For this review, use the dimensioned drawing (mm, ordinates from the lowest corner) and the shaded views. A direction names the side the tool comes from. Coordinates: 2 decimals unless noted, no trailing zeros. Loops run counter-clockwise (first coordinate to the right, second up) from the corner with the lowest first, then second, coordinate; pieces in that order, holes last. Notation, with made-up numbers: (30, 15.5) - (40, 15.5) arc R28 cw to (40, 44.5) - close; hole circle Ø11 at (-24, 68). An arc over 180 degrees is marked (long way). Use a Markdown table: item, result. Add a question column.
1) Add section A-A, the plane z = 11.5. Give the boundary of the cut face in (x, y), and give its area (3 significant figures).
2) Add section D-D, the plane z = 29. Give the boundary of the cut face in (x, y) (3 decimals).
3) The part is to be moulded in two halves that separate along Y. For the marked faces 1, 2, 3 and 4, say which applies: pulls with the +Y half, pulls with the -Y half, needs draft (parallel to the pull), parting line crosses it, or undercut.
4) Clearance check with a flat-ended pin moving along its axis: pin 1 (1.6 mm diameter, centred on x = 25.5, y = 119.5, fed in from +Z). State where the tip first meets the part, or that it passes through.
5) Add section B-B, the plane y = 100.4. Give the boundary of the cut face in (x, z).
6) To check wall thickness, follow L1, parallel to Y at x = 60.5, z = 12; L2, parallel to Z at x = 185, y = 113. State the ranges of each line that lie inside material, in increasing order. Write a range as [from, to].
7) Add section C-C, the plane x = 112.7. Give the boundary of the cut face in (y, z) (3 decimals).
8) For the marked faces 5 and 6, list the 3-axis set-ups (+Z, -Z, +X, -X, +Y, -Y) from which the entire face can be reached by the end or side of a thin tool; tool diameter is ignored.
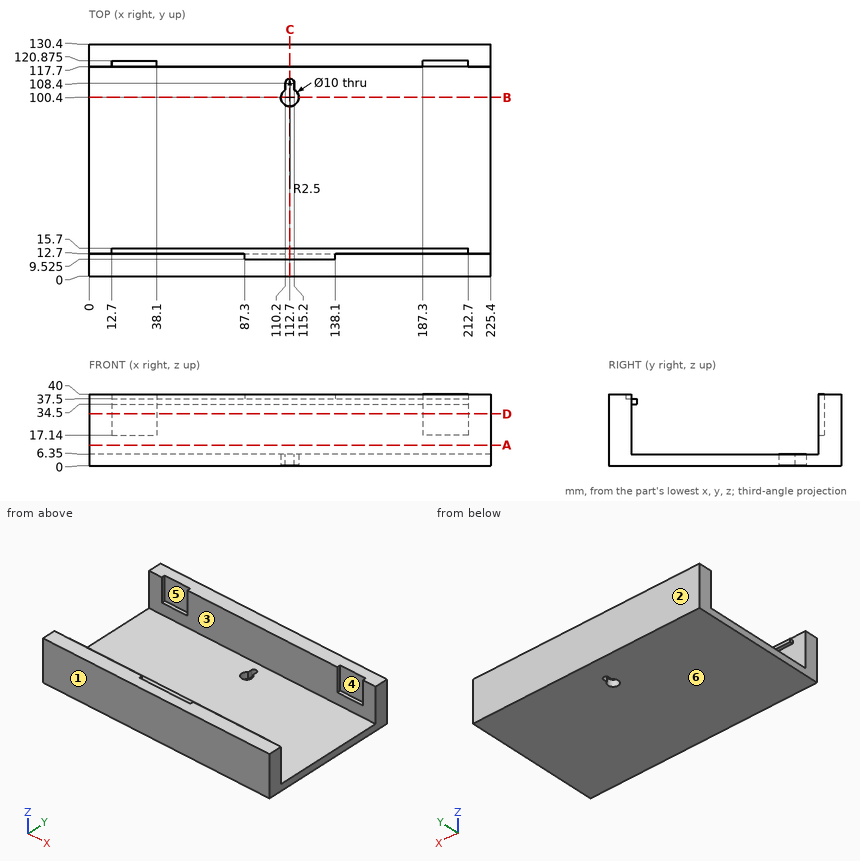
From the geometry:
| question | item | result |
|---|---|---|
| 1 | outline | (0, 0) - (225.4, 0) - (225.4, 12.7) - (0, 12.7) - close; (0, 117.7) - (225.4, 117.7) - (225.4, 130.4) - (0, 130.4) - close |
| 1 | area | 5,730 mm^2 |
| 2 | outline | (0, 0) - (225.4, 0) - (225.4, 12.7) - (0, 12.7) - close; (0, 117.7) - (12.7, 117.7) - (12.7, 120.875) - (38.1, 120.875) - (38.1, 117.7) - (187.3, 117.7) - (187.3, 120.875) - (212.7, 120.875) - (212.7, 117.7) - (225.4, 117.7) - (225.4, 130.4) - (0, 130.4) - close |
| 3 | face 1 | pulls with the -Y half |
| 3 | face 2 | pulls with the +Y half |
| 3 | face 3 | undercut |
| 3 | face 4 | undercut |
| 4 | pin 1 | stops at z = 17.14 |
| 5 | outline | (0, 0) - (107.7, 0) - (107.7, 6.35) - (0, 6.35) - close; (117.7, 0) - (225.4, 0) - (225.4, 6.35) - (117.7, 6.35) - close |
| 6 | L1 | y = [0, 12.7], [117.7, 130.4] |
| 6 | L2 | z = [0, 6.35] |
| 7 | outline | (0, 0) - (95.4, 0) - (95.4, 6.35) - (12.7, 6.35) - (12.7, 34.5) - (15.7, 34.5) - (15.7, 37.5) - (9.525, 37.5) - (9.525, 40) - (0, 40) - close; (110.9, 0) - (130.4, 0) - (130.4, 40) - (117.7, 40) - (117.7, 6.35) - (110.9, 6.35) - close |
| 8 | face 5 | +Z |
| 8 | face 6 | -Z, +X, -X, +Y, -Y |
